The model under review builds one solid part; all positions refer to its coordinate system, in mm. Round coordinates to 2 decimals unless told otherwise and drop trailing zeros. Write each loop counter-clockwise with the first axis right and the second up, starting at its lowest first coordinate (ties: lowest second). Pieces come first, ordered by that corner, then holes. Notation, with made-up numbers: (68.5, 29.5) -> (76.5, 29.5) arc R28 ccw to (76.5, 53.5) -> close; hole circle Ø6 at (50, 64.5). An arc over 180 degrees is marked (long way). Return JSON: item names as keys, results as strings. Group by question number.
1. For line 1 along X through (y, z) = (29, -1.3); line 2 along Y through (x, z) = (20.3, 0.1) (3 decimals); line 3 along Y through (x, z) = (-170.7, -0.6), list the stretches that pass through material, from the lowest coordinate up. Write a range as from..to.
2. Take a section at B-B, the plane x = -67. Write out the cut boundary in (y, z).
3. Clearance check with flat-ended pins moving along their axes: P1, Ø2, axis at x = -157, z = 0, coming from the +Y side; P2, Ø1.5, axis at x = -78.5, z = 0.5, coming from the +Y side; P3, Ø3.5, axis at x = -141, y = 23.48, coming from the +Z side; P4, Ø3, axis at x = 20.3, y = -22.6, coming from the +Z side. State where each tip first meets the part, or that it passes through.
4. Take a section at A-A, the plane y = 0. Write out the cut boundary in (x, z), then the cut area to 3 significant figures.
5. Take a section at C-C, the plane z = -1.2. Give the number of separate pieces and of enclosed holes in the cut face, then the cut area to 3 significant figures.
from build123d import *

# Parameters (mm, degrees)
SKETCH_1_W                   = 200
SKETCH_1_H                   = 53.2
SKETCH_1_R                   = 6.5
SKETCH_1_R_2                 = 2.025
EXTRUDE_1_DEPTH              = 2
SKETCH_2_R                   = 20
CUT_EXTRUDE_1_DEPTH          = 5
CUT_EXTRUDE_2_DEPTH          = 10
SKETCH_4_R                   = 1.1
CUT_EXTRUDE_3_DEPTH          = 10
SKETCH_5_W                   = 70
SKETCH_5_H                   = 13.4
SKETCH_5_R                   = 1.6
EXTRUDE_2_DEPTH              = 4
EXTRUDE_3_DEPTH              = 4
SKETCH_7_W                   = 12.3
SKETCH_7_H                   = 15.2
CUT_EXTRUDE_4_DEPTH          = 10
CUT_EXTRUDE_5_DEPTH          = 10
EXTRUDE_1_2_DEPTH            = 4
SKETCH_10_R                  = 1.1
CUT_EXTRUDE_6_DEPTH          = 4
FILLET_1_R                   = 2
CUT_EXTRUDE_7_DEPTH          = 4
FILLET_2_R                   = 2
SKETCH_12_R                  = 1.55
CUT_EXTRUDE_8_DEPTH          = 10
HOLE_WIZARD_M3_1_D           = 3.4
HOLE_WIZARD_M3_1_CSINK_D     = 6.3
HOLE_WIZARD_M3_1_CSINK_ANGLE = 90
SKETCH_16_W                  = 6
SKETCH_16_H                  = 4.5
CUT_EXTRUDE_9_DEPTH          = 10
FILLET_3_R                   = 1


with BuildPart() as part:
    # 草图1 → Extrude 1 (new, symmetric)
    with BuildSketch(Plane.XY):
        with Locations((-75.7, 0)):
            Rectangle(SKETCH_1_W, SKETCH_1_H)
        Circle(SKETCH_1_R, mode=Mode.SUBTRACT)
        with Locations((20.3, 22.6)):
            Circle(SKETCH_1_R_2, mode=Mode.SUBTRACT)
        with Locations((20.3, 12.6)):
            Circle(SKETCH_1_R_2, mode=Mode.SUBTRACT)
        with Locations((20.3, -12.6)):
            Circle(SKETCH_1_R_2, mode=Mode.SUBTRACT)
        with Locations((20.3, -22.6)):
            Circle(SKETCH_1_R_2, mode=Mode.SUBTRACT)
    extrude(amount=EXTRUDE_1_DEPTH, both=True)

    # 草图2 → 切除-拉伸1 (cut)
    with BuildSketch(Plane.XY.offset(2)):
        with Locations((-148, 0)):
            Circle(SKETCH_2_R)
    extrude(amount=-CUT_EXTRUDE_1_DEPTH, mode=Mode.SUBTRACT)

    # 草图3 → 切除-拉伸2 (cut)
    with BuildSketch(Plane.XY.offset(2)):
        with BuildLine():
            Line((-136.21195189, -26.6), (-139.272801212, -12.199836119))
            ThreePointArc((-139.272801212, -12.199836119), (-151.628828434, -14.554435894), (-161.43313529, -6.674644281))
            Line((-161.43313529, -6.674644281), (-175.7, -23.677231554))
            Line((-175.7, -23.677231554), (-175.7, -26.6))
            Line((-175.7, -26.6), (-136.21195189, -26.6))
        make_face()
    extrude(amount=-CUT_EXTRUDE_2_DEPTH, mode=Mode.SUBTRACT)

    # 草图4 → 切除-拉伸3 (cut)
    with BuildSketch(Plane.XY.offset(2)):
        with Locations((-141, 23.478713764)):
            Circle(SKETCH_4_R)
        with Locations((-131.166837432, -17.801534708)):
            Circle(SKETCH_4_R)
        with Locations((-171.833162568, -5.677179055)):
            Circle(SKETCH_4_R)
    extrude(amount=-CUT_EXTRUDE_3_DEPTH, mode=Mode.SUBTRACT)

    # 草图5 → 凸台-拉伸2 (add)
    with BuildSketch(Plane.XY.offset(2)):
        with Locations((-140.7, 33.3)):
            Rectangle(SKETCH_5_W, SKETCH_5_H)
        with Locations((-170.7, 37)):
            Circle(SKETCH_5_R, mode=Mode.SUBTRACT)
        with Locations((-150.7, 37)):
            Circle(SKETCH_5_R, mode=Mode.SUBTRACT)
    extrude(amount=-EXTRUDE_2_DEPTH)

    # 草图6 → 凸台-拉伸3 (add)
    with BuildSketch(Plane.XY.offset(2)):
        Polygon((-175.7, 40), (-178.7, 40), (-178.7, -27.252492331), (-175.7, -23.677231554), align=None)
    extrude(amount=-EXTRUDE_3_DEPTH)

    # 草图7 → 切除-拉伸4 (cut)
    with BuildSketch(Plane.XY.offset(2)):
        with Locations((18.15, 0)):
            Rectangle(SKETCH_7_W, SKETCH_7_H)
        with BuildLine():
            Line((15.3, -11.1), (5.748043145, -11.1))
            ThreePointArc((5.748043145, -11.1), (0, -12.5), (-5.748043145, -11.1))
            Line((-5.748043145, -11.1), (-9, -11.1))
            Line((-9, -11.1), (-9, -20.6))
            Line((-9, -20.6), (15.3, -20.6))
            Line((15.3, -20.6), (15.3, -11.1))
        make_face()
        with BuildLine():
            ThreePointArc((-5.748043145, 11.1), (0, 12.5), (5.748043145, 11.1))
            Line((5.748043145, 11.1), (15.3, 11.1))
            Line((15.3, 11.1), (15.3, 20.6))
            Line((15.3, 20.6), (-9, 20.6))
            Line((-9, 20.6), (-9, 11.1))
            Line((-9, 11.1), (-5.748043145, 11.1))
        make_face()
    extrude(amount=-CUT_EXTRUDE_4_DEPTH, mode=Mode.SUBTRACT)

    # 草图8 → 切除-拉伸5 (cut)
    with BuildSketch(Plane.XY.offset(2)):
        with BuildLine():
            Line((-17, -20.6), (-129.782151609, -20.6))
            ThreePointArc((-129.782151609, -20.6), (-120.5, 0), (-129.782151609, 20.6))
            Line((-129.782151609, 20.6), (-17, 20.6))
            Line((-17, 20.6), (-17, -20.6))
        make_face()
    extrude(amount=-CUT_EXTRUDE_5_DEPTH, mode=Mode.SUBTRACT)

    # 草图9 → Extrude 1 2 (add)
    with BuildSketch(Plane.XY.offset(2)):
        Polygon((-16.056398464, -18.016956032), (-128.838550073, 23.183043968), (-130.725753145, 18.016956032), (-17.943601536, -23.183043968), align=None)
        Polygon((-17.943601536, 23.183043968), (-130.725753145, -18.016956032), (-128.838550073, -23.183043968), (-16.056398464, 18.016956032), align=None)
    extrude(amount=-EXTRUDE_1_2_DEPTH)

    # 草图10 → 切除-拉伸6 (cut)
    with BuildSketch(Plane.XY.offset(2)):
        with Locations((-131.166837432, -17.801534708)):
            Circle(SKETCH_10_R)
    extrude(amount=-CUT_EXTRUDE_6_DEPTH, mode=Mode.SUBTRACT)

    # 圆角1
    fillet_1_edges = [part.edges().sort_by_distance(p)[0] for p in [
        (-178.7, -27.252492331, 0),
        (-178.7, 40, 0),
        (24.3, -7.6, 0),
        (24.3, 7.6, 0),
        (-5.748043145, -11.1, 0),
        (5.748043145, -11.1, 0),
        (15.3, -11.1, 0),
        (15.3, -20.6, 0),
        (-9, -20.6, 0),
        (-9, -11.1, 0),
        (5.748043145, 11.1, 0),
        (-5.748043145, 11.1, 0),
        (-9, 11.1, 0),
        (-9, 20.6, 0),
        (15.3, 20.6, 0),
        (15.3, 11.1, 0),
        (12, -7.6, 0),
        (12, 7.6, 0),
        (-25.014505818, 20.6, 0),
        (-121.767645791, 20.6, 0),
        (-125.787682754, -16.213049144, 0),
        (-125.787682754, 16.213049144, 0),
        (-121.767645791, -20.6, 0),
        (-25.014505818, -20.6, 0),
        (-17, 17.672252701, 0),
        (-17, -17.672252701, 0),
        (-65.376569986, 0, 0),
        (-73.391075804, -2.927747299, 0),
        (-81.405581623, 0, 0),
        (-73.391075804, 2.927747299, 0),
        (-164.85987264, -10.758470828, 0),
        (-138.16441215, -17.414396677, 0),
        (-136.21195189, -26.6, 0),
        (24.3, 26.6, 0),
        (24.3, -26.6, 0),
        (-105.7, 40, 0),
        (-105.7, 26.6, 0),
    ]]
    fillet(fillet_1_edges, radius=FILLET_1_R)

    # 草图11 → 切除-拉伸7 (cut)
    with BuildSketch(Plane.XY.offset(2)):
        with BuildLine():
            Line((-110.7, 26.6), (-110.7, 33))
            Line((-110.7, 33), (-145, 33))
            Line((-145, 33), (-145, 27.335873866))
            ThreePointArc((-145, 27.335873866), (-140.342710532, 26.412419768), (-135.913677776, 24.701635879))
            ThreePointArc((-135.913677776, 24.701635879), (-123.049148512, 22.228227917), (-110.7, 26.6))
        make_face()
        with BuildLine():
            Line((-173.7, 33), (-151, 33))
            Line((-151, 33), (-151, 27.335873866))
            ThreePointArc((-151, 27.335873866), (-164.82036316, 21.756042452), (-173.7, 9.785703858))
            Line((-173.7, 9.785703858), (-173.7, 33))
        make_face()
    extrude(amount=-CUT_EXTRUDE_7_DEPTH, mode=Mode.SUBTRACT)

    # 圆角2
    fillet_2_edges = [part.edges().sort_by_distance(p)[0] for p in [
        (-110.7, 26.6, 0),
        (-145, 27.335873866, 0),
        (-145, 33, 0),
        (-110.7, 33, 0),
        (-173.7, 9.785703858, 0),
        (-173.7, 33, 0),
        (-151, 33, 0),
        (-151, 27.335873866, 0),
    ]]
    fillet(fillet_2_edges, radius=FILLET_2_R)

    # 草图12 → 切除-拉伸8 (cut)
    with BuildSketch(Plane.XY.offset(2)):
        with Locations((-25, -22.6)):
            Circle(SKETCH_12_R)
    extrude(amount=-CUT_EXTRUDE_8_DEPTH, mode=Mode.SUBTRACT)

    # M3 锥坑平头螺钉的锥形沉头孔1 (through all)
    with Locations(Plane(origin=(0, 0, -2), x_dir=(-1, 0, 0), z_dir=(0, 0, -1))):
        with Locations((25, -22.6)):
            CounterSinkHole(HOLE_WIZARD_M3_1_D / 2, HOLE_WIZARD_M3_1_CSINK_D / 2, counter_sink_angle=HOLE_WIZARD_M3_1_CSINK_ANGLE)

    # 草图16 → 切除-拉伸9 (cut)
    with BuildSketch(Plane.XY.offset(2)):
        with Locations((-120.7, 37.75)):
            Rectangle(SKETCH_16_W, SKETCH_16_H)
        with Locations((-156.7, 37.75)):
            Rectangle(SKETCH_16_W, SKETCH_16_H)
    extrude(amount=-CUT_EXTRUDE_9_DEPTH, mode=Mode.SUBTRACT)

    # 圆角3
    fillet_3_edges = [part.edges().sort_by_distance(p)[0] for p in [
        (-153.7, 40, 0),
        (-159.7, 40, 0),
        (-117.7, 40, 0),
        (-123.7, 40, 0),
        (-117.7, 35.5, 0),
        (-123.7, 35.5, 0),
        (-153.7, 35.5, 0),
        (-159.7, 35.5, 0),
    ]]
    fillet(fillet_3_edges, radius=FILLET_3_R)


solid = part.part
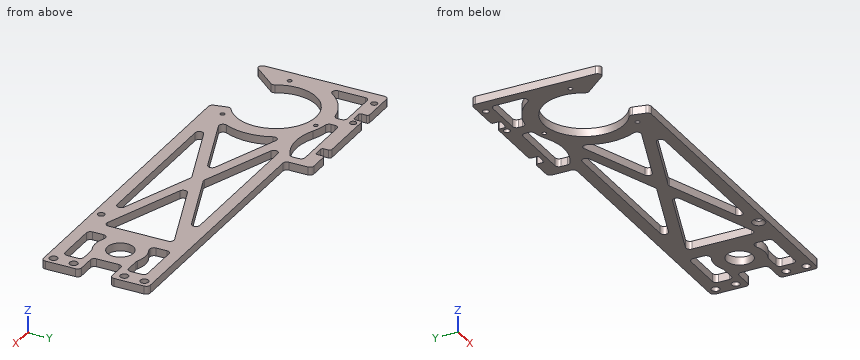
Output:
{
 "1": {"line 1": "x = -178.7..-173.7, -151..-145, -110.7..-105.7", "line 2": "y = -26.6..-24.625, -20.575..-14.625, -10.575..-7.6, 7.6..10.575, 14.625..20.575, 24.625..26.6", "line 3": "y = -17.72..15.83, 33..35.4, 38.6..40"},
 "2": {"outline": "(-26.6, -2) -> (-20.6, -2) -> (-20.6, 2) -> (-26.6, 2) -> close; (-5.26, -2) -> (5.26, -2) -> (5.26, 2) -> (-5.26, 2) -> close; (20.6, -2) -> (26.6, -2) -> (26.6, 2) -> (20.6, 2) -> close"},
 "3": {"P1": "stops at y = 35.5", "P2": "stops at y = 26.6", "P3": "stops at z = 2", "P4": "passes through"},
 "4": {"outline": "(-178.7, -2) -> (-168, -2) -> (-168, 2) -> (-178.7, 2) -> close; (-128, -2) -> (-120.5, -2) -> (-120.5, 2) -> (-128, 2) -> close; (-85.23, -2) -> (-61.55, -2) -> (-61.55, 2) -> (-85.23, 2) -> close; (-17, -2) -> (-6.5, -2) -> (-6.5, 2) -> (-17, 2) -> close; (6.5, -2) -> (12, -2) -> (12, 2) -> (6.5, 2) -> close", "area": "232 mm^2"},
 "5": {"separate pieces": "1", "enclosed holes": "19", "area": "5,650 mm^2"}
}
